Answer from the drawing. Dimensions are ordinates in mm from the lowest x, y and z of the part. A direction names the side the tool comes from. Give positions to 0.01 mm unless a question says otherwise; leave off trailing zeros. Order: outer loops, then holes, each group sorted by start corner. A loop starts at its lowest first (then second) coordinate and runs counter-clockwise, first axis right, second up.
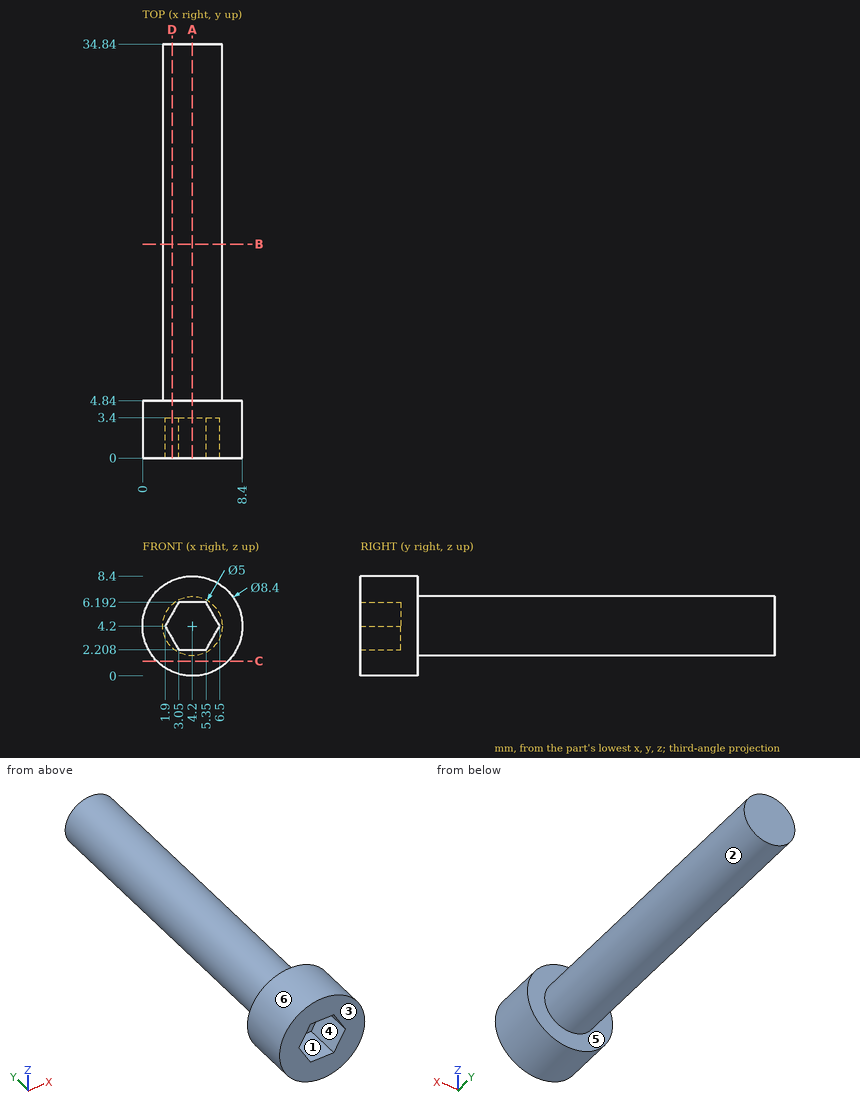
1) The part is cut by section C-C on z = 1.25. Determine the outline of the cut face in (x, y).
Final values:
outline: (1.21, 0) - (7.19, 0) - (7.19, 4.84) - (1.21, 4.84) - close
2) The part is cut by section B-B on y = 18. Determine the outline of the cut face in (x, z), and give its area (3 significant figures).
Final values:
outline: circle Ø5 at (4.2, 4.2)
area: 19.6 mm2
3) Consider L1, parallel to Y at x = 2.25, z = 1.5; L2, parallel to Y at x = 3.5, z = 2.5; L3, parallel to X at y = 14, z = 4.25. Determine where each line is inside the solid, lowest interval first.
Final values:
L1: y = 0 to 4.84
L2: y = 3.4 to 34.84
L3: x = 1.7 to 6.7
4) The part is cut by section A-A on x = 4.2. Determine the outline of the cut face in (y, z).
Final values:
outline: (0, 0) - (4.84, 0) - (4.84, 1.7) - (34.84, 1.7) - (34.84, 6.7) - (4.84, 6.7) - (4.84, 8.4) - (0, 8.4) - (0, 6.19) - (3.4, 6.19) - (3.4, 2.21) - (0, 2.21) - close
5) The part is cut by section D-D on x = 2.5. Determine the outline of the cut face in (y, z).
Final values:
outline: (0, 0.36) - (4.84, 0.36) - (4.84, 2.37) - (34.84, 2.37) - (34.84, 6.03) - (4.84, 6.03) - (4.84, 8.04) - (0, 8.04) - (0, 5.24) - (3.4, 5.24) - (3.4, 3.16) - (0, 3.16) - close
6) A tool of negligible diameter and unlimited length cuts with its end or side. For the marked faces 5 and 6, from which of +Z, -Z, +X, -X, +Y, -Y can it reach the whole face along a straight path? Write none if from no direction.
Final values:
face 5: +Y
face 6: +Y, -Y
7) For a pull along Z with two mould halves and no side action, classify the marked faces 1, 2, 3 and 4 as released by +Z, released by -Z, zero draft, split by the parting line, or undercut.
Final values:
face 1: undercut
face 2: split by the parting line
face 3: zero draft
face 4: undercut
8) Given pin 1 (2 mm diameter, centred on x = 2.5, z = 2, fed in from -Y); pin 2 (1 mm diameter, centred on x = 3.5, y = 6, fed in from +Z); pin 3 (3 mm diameter, centred on y = 15, z = 5, fed in from -X); pin 4 (3 mm diameter, centred on y = 12, z = 1, fed in from -X), each flat-ended and moving along its own axis, determine where each tip first touches the part or whether it passes through.
Final values:
pin 1: stops at y = 0
pin 2: stops at z = 6.69
pin 3: stops at x = 1.7
pin 4: stops at x = 2.37
